Here's how the part is built. I have some questions about the finished solid (model axes, mm). Face numbers are marked on the shaded views. A direction names the side the tool comes from. Give positions to 0.01 mm unless a question says otherwise; leave off trailing zeros. Write each loop counter-clockwise with the first axis right and the second up, starting at its lowest first coordinate (ties: lowest second). Pieces come first, ordered by that corner, then holes. Notation, with made-up numbers: (69, 47) - (107, 47) arc R30 cw to (107, 79) - close; hole circle Ø5 at (65.5, 57.5). An arc over 180 degrees is marked (long way). Write each question's results on one line, items separated by ' | '. Start each with the question number.
Item 1: Suppose I cut it at A-A on x = 0. List the corners of the cut face in (y, z) for me, then the cut area to 3 significant figures.
Item 2: We'd pull the mould along X, two halves only. Please class the marked faces 1, 2 and 3: +X half, -X half, draft (parallel to the pull), parting line (faces both ways), or undercut.
Item 3: Which directions (+Z, -Z, +X, -X, +Y, -Y) give clear straight access to the entire face, cutting with the end or side of a thin tool? Please do the marked faces 4 and 5.
Item 4: Will these pins go through, and if not, where does the flat tip stop? P1, Ø5, axis at x = 13.5, y = -1.5, coming from the +Z side; P2, Ø3, axis at x = 9.5, y = 19, coming from the +Z side.
Item 5: Suppose I cut it at B-B on z = -5.25. List the corners of the cut face in (x, y) for me.
Item 6: Suppose I cut it at C-C on x = 9.5. List the corners of the cut face in (y, z) for me, then the cut area to 3 significant figures.
Item 7: Please list where these lines run through material, in increasing order: line 1 along Y through (x, z) = (24.5, -10); line 2 along Y through (x, z) = (0, -4.5); line 3 along X through (y, z) = (0, -5).
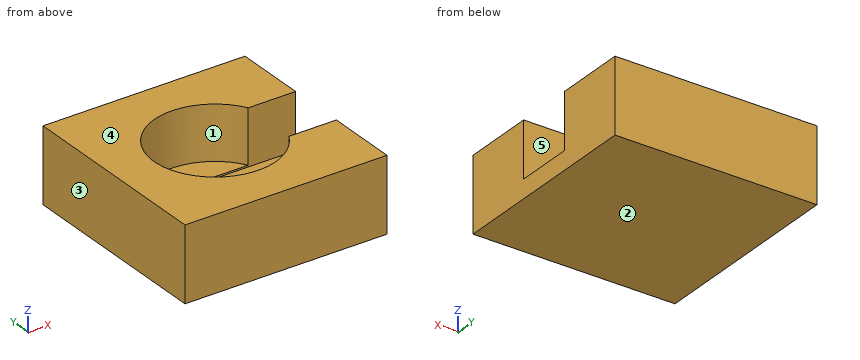
```python
from build123d import *

# Parameters (mm, degrees)
F0_W     = 60
F0_H     = 60
F1_DEPTH = 22
F2_R     = 18.1
F3_DEPTH = 16
F4_W     = 17.230908
F4_H     = 16.499999
F5_DEPTH = 25


with BuildPart() as f1:
    # F0 (on Top) → F1 (new body)
    with BuildSketch(Plane.XY):
        Rectangle(F0_W, F0_H)
    extrude(amount=-F1_DEPTH)

    # F2 (on face) → F3 (cut)
    with BuildSketch(Plane.XY):
        Circle(F2_R)
    extrude(amount=-F3_DEPTH, mode=Mode.SUBTRACT)

    # F4 (on face) → F5 (cut)
    with BuildSketch(Plane.YZ.offset(30)):
        with Locations((0, -8.249999)):
            Rectangle(F4_W, F4_H)
    extrude(amount=-F5_DEPTH, mode=Mode.SUBTRACT)


solid = f1.part
```
Checked values:
1) outline: (-30, -22) - (30, -22) - (30, 0) - (18.1, 0) - (18.1, -16) - (-18.1, -16) - (-18.1, 0) - (-30, 0) - close | area: 741 mm^2
2) face 1: undercut | face 2: draft | face 3: -X half
3) face 4: +Z, +X, -X, +Y, -Y | face 5: +Z, +X
4) P1: stops at z = -16.5 | P2: stops at z = 0
5) outline: (-30, -30) - (30, -30) - (30, -8.62) - (15.92, -8.62) arc R18.1 cw (long way) to (15.92, 8.62) - (30, 8.62) - (30, 30) - (-30, 30) - close
6) outline: (-30, -22) - (30, -22) - (30, 0) - (15.41, 0) - (15.41, -16) - (8.62, -16) - (8.62, -16.5) - (-8.62, -16.5) - (-8.62, -16) - (-15.41, -16) - (-15.41, 0) - (-30, 0) - close | area: 818 mm^2
7) line 1: y = -30 to -8.62, 8.62 to 30 | line 2: y = -30 to -18.1, 18.1 to 30 | line 3: x = -30 to -18.1
